```python
from build123d import *

# Parameters (mm, degrees)
ESQUISSE1_R        = 9.739786638
BOSS_EXTRU_1_DEPTH = 5.5
ESQUISSE2_R        = 9.739786638
ESQUISSE2_R_2      = 1.4
BOSS_EXTRU_2_DEPTH = 0.5
CHANFREIN1_SIZE    = 0.2
BOSS_EXTRU_3_START = -5.5
BOSS_EXTRU_3_DEPTH = 5.5
BOSS_EXTRU_4_START = 42
BOSS_EXTRU_4_DEPTH = 42
BOSS_EXTRU_5_DEPTH = 22
BOSS_EXTRU_6_DEPTH = 46.25
ESQUISSE7_W        = 6
ESQUISSE7_H        = 17.089185867
BOSS_EXTRU_7_DEPTH = 23


with BuildPart() as part:
    # Esquisse1 → Boss.-Extru.1 (new body)
    with BuildSketch(Plane.XY):
        with Locations((-10.25, -10)):
            Circle(ESQUISSE1_R)
        with BuildLine():
            Line((-5.751675839, -9.877200395), (-6.833750507, -9.782531128))
            Line((-6.833750507, -9.782531128), (-6.949445107, -9.126394451))
            Line((-6.949445107, -9.126394451), (-5.953521963, -8.661987862))
            ThreePointArc((-5.953521963, -8.661987862), (-6.006634107, -8.502052772), (-6.065697468, -8.344218516))
            Line((-6.065697468, -8.344218516), (-7.138261768, -8.631611254))
            Line((-7.138261768, -8.631611254), (-7.47139109, -8.054614344))
            Line((-7.47139109, -8.054614344), (-6.678798898, -7.262022153))
            ThreePointArc((-6.678798898, -7.262022153), (-6.782621037, -7.131675902), (-6.891198054, -7.005263035))
            Line((-6.891198054, -7.005263035), (-7.818046533, -7.654249327))
            Line((-7.818046533, -7.654249327), (-8.328430264, -7.225986526))
            Line((-8.328430264, -7.225986526), (-7.847635402, -6.194918616))
            ThreePointArc((-7.847635402, -6.194918616), (-7.988951343, -6.109285545), (-8.133315872, -6.028898352))
            Line((-8.133315872, -6.028898352), (-8.791112727, -6.968329619))
            Line((-8.791112727, -6.968329619), (-9.417191057, -6.740455742))
            Line((-9.417191057, -6.740455742), (-9.317216173, -5.597737589))
            ThreePointArc((-9.317216173, -5.597737589), (-9.478728542, -5.566588183), (-9.641271425, -5.541362369))
            Line((-9.641271425, -5.541362369), (-9.940094206, -6.656584169))
            Line((-9.940094206, -6.656584169), (-10.606352849, -6.656584169))
            Line((-10.606352849, -6.656584169), (-10.903477232, -5.547700874))
            ThreePointArc((-10.903477232, -5.547700874), (-11.065761738, -5.574558464), (-11.226956242, -5.607329229))
            Line((-11.226956242, -5.607329229), (-11.126406846, -6.756614081))
            Line((-11.126406846, -6.756614081), (-11.752485176, -6.984487958))
            Line((-11.752485176, -6.984487958), (-12.406540122, -6.050400691))
            ThreePointArc((-12.406540122, -6.050400691), (-12.550096477, -6.132241451), (-12.690551241, -6.219297732))
            Line((-12.690551241, -6.219297732), (-12.206963835, -7.256354271))
            Line((-12.206963835, -7.256354271), (-12.717347566, -7.684617071))
            Line((-12.717347566, -7.684617071), (-13.638885709, -7.039349117))
            ThreePointArc((-13.638885709, -7.039349117), (-13.74618945, -7.166864047), (-13.848697947, -7.298264801))
            Line((-13.848697947, -7.298264801), (-13.051434053, -8.095528695))
            Line((-13.051434053, -8.095528695), (-13.384563375, -8.672525605))
            Line((-13.384563375, -8.672525605), (-14.450903238, -8.3868007))
            ThreePointArc((-14.450903238, -8.3868007), (-14.508366703, -8.545244687), (-14.559856563, -8.705729393))
            Line((-14.559856563, -8.705729393), (-13.557961929, -9.172920534))
            Line((-13.557961929, -9.172920534), (-13.673656528, -9.829057211))
            Line((-13.673656528, -9.829057211), (-14.74934404, -9.923167674))
            ThreePointArc((-14.74934404, -9.923167674), (-14.749021481, -10.093838761), (-14.74222728, -10.264374865))
            Line((-14.74222728, -10.264374865), (-13.665452724, -10.358580432))
            Line((-13.665452724, -10.358580432), (-13.549758125, -11.014717109))
            Line((-13.549758125, -11.014717109), (-14.506309194, -11.460764198))
            ThreePointArc((-14.506309194, -11.460764198), (-14.447094307, -11.623083293), (-14.381691786, -11.78300953))
            Line((-14.381691786, -11.78300953), (-13.360941463, -11.509500306))
            Line((-13.360941463, -11.509500306), (-13.027812142, -12.086497216))
            Line((-13.027812142, -12.086497216), (-13.758807936, -12.817493011))
            ThreePointArc((-13.758807936, -12.817493011), (-13.646852578, -12.951506829), (-13.529782028, -13.081076086))
            Line((-13.529782028, -13.081076086), (-12.681156698, -12.486862233))
            Line((-12.681156698, -12.486862233), (-12.170772967, -12.915125033))
            Line((-12.170772967, -12.915125033), (-12.600738895, -13.837189942))
            ThreePointArc((-12.600738895, -13.837189942), (-12.448909121, -13.926168447), (-12.293716433, -14.009142444))
            Line((-12.293716433, -14.009142444), (-11.708090504, -13.172781941))
            Line((-11.708090504, -13.172781941), (-11.082012174, -13.400655818))
            Line((-11.082012174, -13.400655818), (-11.169878896, -14.404977051))
            ThreePointArc((-11.169878896, -14.404977051), (-10.996236031, -14.437694422), (-10.821442589, -14.463569577))
            Line((-10.821442589, -14.463569577), (-10.559109026, -13.48452739))
            Line((-10.559109026, -13.48452739), (-9.892850383, -13.48452739))
            Line((-9.892850383, -13.48452739), (-9.632173683, -14.457386077))
            ThreePointArc((-9.632173683, -14.457386077), (-9.45766281, -14.42969545), (-9.284373537, -14.395175256))
            Line((-9.284373537, -14.395175256), (-9.372796385, -13.384497479))
            Line((-9.372796385, -13.384497479), (-8.746718055, -13.156623602))
            Line((-8.746718055, -13.156623602), (-8.164782025, -13.987714383))
            ThreePointArc((-8.164782025, -13.987714383), (-8.010469052, -13.903139907), (-7.859580663, -13.812596936))
            Line((-7.859580663, -13.812596936), (-8.292239396, -12.884757289))
            Line((-8.292239396, -12.884757289), (-7.781855665, -12.456494489))
            Line((-7.781855665, -12.456494489), (-6.938532496, -13.046995729))
            ThreePointArc((-6.938532496, -13.046995729), (-6.822819391, -12.916236114), (-6.712266113, -12.78108593))
            Line((-6.712266113, -12.78108593), (-7.447769178, -12.045582865))
            Line((-7.447769178, -12.045582865), (-7.114639857, -11.468585954))
            Line((-7.114639857, -11.468585954), (-6.100183444, -11.740408731))
            ThreePointArc((-6.100183444, -11.740408731), (-6.036436962, -11.579837499), (-5.978900904, -11.416937723))
            Line((-5.978900904, -11.416937723), (-6.941241303, -10.968191026))
            Line((-6.941241303, -10.968191026), (-6.825546704, -10.312054348))
            Line((-6.825546704, -10.312054348), (-5.755303948, -10.21842024))
            ThreePointArc((-5.755303948, -10.21842024), (-5.750254354, -10.04784472), (-5.751675839, -9.877200395))
        make_face(mode=Mode.SUBTRACT)
    extrude(amount=BOSS_EXTRU_1_DEPTH)

    # Esquisse2 → Boss.-Extru.2 (add)
    with BuildSketch(Plane.XY.offset(5.5)):
        with Locations((-10.25, -10)):
            Circle(ESQUISSE2_R)
        with Locations((-10.249601616, -10.07055578)):
            Circle(ESQUISSE2_R_2, mode=Mode.SUBTRACT)
    extrude(amount=BOSS_EXTRU_2_DEPTH)

    # Chanfrein1
    chanfrein1_edges = [part.edges().sort_by_distance(p)[0] for p in [
        (-11.649601616, -10.07055578, 6),
    ]]
    chamfer(chanfrein1_edges, length=CHANFREIN1_SIZE)

    # Esquisse3 → Boss.-Extru.3 (add)
    with BuildSketch(Plane.XY.offset(6).offset(BOSS_EXTRU_3_START)):
        with BuildLine():
            Line((-10.25, -0.260213362), (39.75, -0.260213362))
            Line((39.75, -0.260213362), (39.75, -19.739786638))
            Line((39.75, -19.739786638), (-10.25, -19.739786638))
            ThreePointArc((-10.25, -19.739786638), (-19.989786638, -10), (-10.25, -0.260213362))
        make_face()
        with BuildLine():
            Line((33.837373972, -17.739786638), (-10.25, -17.739786638))
            ThreePointArc((-10.25, -17.739786638), (-17.989786638, -10), (-10.25, -2.260213362))
            Line((-10.25, -2.260213362), (33.837373972, -2.260213362))
            ThreePointArc((33.837373972, -2.260213362), (30.010213362, -10), (33.837373972, -17.739786638))
        make_face(mode=Mode.SUBTRACT)
    extrude(amount=BOSS_EXTRU_3_DEPTH)

    # Esquisse4 → Boss.-Extru.4 (add)
    with BuildSketch(Plane(origin=(0, 0, 0.5), x_dir=(-1, 0, 0), z_dir=(0, 0, -1)).offset(BOSS_EXTRU_4_START)):
        with BuildLine():
            Line((-39.75, -0.260213362), (-39.75, -19.739786638))
            ThreePointArc((-39.75, -19.739786638), (-30.010213362, -10), (-39.75, -0.260213362))
        make_face()
    extrude(amount=-BOSS_EXTRU_4_DEPTH)

    # Esquisse5 → Boss.-Extru.5 (add)
    with BuildSketch(Plane(origin=(39.75, 0, 0), x_dir=(0, 0, -1), z_dir=(1, 0, 0))):
        Polygon((34.25, -0.260213362), (34.25, -17.347570489), (39.5, -17.347570489), (41.5, -17.347570489), (41.5, -0.260213362), align=None)
    extrude(amount=BOSS_EXTRU_5_DEPTH)

    # Esquisse6 → Boss.-Extru.6 (add)
    with BuildSketch(Plane.XY.offset(-34.25)):
        Polygon((61.75, -0.260213362), (59.5, -0.260213362), (59.75, -17.347570489), (61.75, -17.347570489), align=None)
    extrude(amount=BOSS_EXTRU_6_DEPTH)

    # Esquisse7 → Boss.-Extru.7 (add)
    with BuildSketch(Plane(origin=(59.483460022, 0.870284673, 0), x_dir=(0, 0, 1), z_dir=(-0.9998929884849062, -0.014629134585590956, 0))):
        with Locations((9, -9.675211958)):
            Rectangle(ESQUISSE7_W, ESQUISSE7_H)
    extrude(amount=BOSS_EXTRU_7_DEPTH)


solid = part.part
```
Source: CAD feature listing. Evaluate the final solid. Frame: model axes, mm. A direction names the side the tool comes from. Coordinates: 2 decimals unless noted, no trailing zeros. Loops run counter-clockwise (first coordinate to the right, second up) from the corner with the lowest first, then second, coordinate; pieces in that order, holes last. Notation, with made-up numbers: (-15, -23) -> (-8, -23) arc R13 ccw to (-8, -6) -> close; hole circle Ø8 at (-0.75, -1.75). An arc over 180 degrees is marked (long way). One line per item, written item: value. Start each with the question number.
Q1. Section query B-B, the plane x = 5. Return the cut outline in (y, z), and give its area (3 significant figures).
Q2. Section query C-C, the plane z = -18. Return the cut outline in (x, y).
Q3. Section query D-D, the plane z = 4. Give the number of separate pieces and of enclosed holes in the cut face, and give its area (3 significant figures).
Q4. Set-up query: faces 4 (the face through (54, -17.348, -35)), 5 (the face through (-10, -14, 0)), 6 (the face through (15, -1, 0.5)). Return all of +Z, -Z, +X, -X, +Y, -Y with unobstructed straight access to the full face (end or side cutting, diameter ignored); none if empty.
Q5. Contact query for flat-ended pins moving along their axis: P1, Ø4.5, axis at x = -10.5, y = -9.5, coming from the -Z side; P2, Ø3, axis at x = 31, z = -19, coming from the +Y side; P3, Ø1, axis at x = 24.5, y = -1.5, coming from the -Z side; P4, Ø11, axis at x = 51.5, z = -15, coming from the -Y side. Output: stop coordinate, or through.
Q6. Section query A-A, the plane y = -3.25. Return the cut outline in (x, z), and give its area (3 significant figures).
Q7. Mould query, pull axis Z, two halves, no side actions, for faces 1 (the face through (50, -9, -34.25)), 2 (the face through (15, -19, 0.5)), 3 (the face through (15, -17.74, 3)). Classes: pulls with the +Z half, pulls with the -Z half, needs draft (parallel to the pull), parting line crosses it, or undercut.
Q8. Line query: line 1 along Y through (x, z) = (22.5, 5.5); line 2 along X through (y, z) = (-14.5, 4.5); line 3 along Z through (x, y) = (53.5, -4). Output: solid intervals per line, ascending.
Results:
1. outline: (-19.74, 0.5) -> (-17.74, 0.5) -> (-17.74, 6) -> (-19.74, 6) -> close; (-2.26, 0.5) -> (-0.26, 0.5) -> (-0.26, 6) -> (-2.26, 6) -> close
1. area: 22.0 mm^2
2. outline: (39.75, -19.74) -> (39.75, -0.26) arc R9.74 ccw to start; (59.5, -0.26) -> (59.75, -17.35) -> (61.75, -17.35) -> (61.75, -0.26) -> close
3. separate pieces: 2
3. enclosed holes: 2
3. area: 606 mm^2
4. face 4: -Z, +X, -Y
4. face 5: -Z, -X, +Y, -Y
4. face 6: -Z, +Y
5. P1: z = 5.5
5. P2: y = -3.5
5. P3: z = 0.5
5. P4: through
6. outline: (-17.27, 0) -> (-3.23, 0) -> (-3.23, 6) -> (-17.27, 6) -> close; (32.73, -41.5) -> (61.75, -41.5) -> (61.75, 12) -> (36.54, 12) -> (36.54, 6) -> (32.73, 6) -> close; hole (39.75, -34.25) -> (59.54, -34.25) -> (59.54, 6) -> (39.75, 6) -> close
6. area: 817 mm^2
7. face 1: undercut
7. face 2: pulls with the -Z half
7. face 3: needs draft
8. line 1: -19.74 to -17.74, -2.26 to -0.26
8. line 2: -18.89 to -1.61, 31.11 to 39.75, 59.71 to 61.75
8. line 3: -41.5 to -34.25, 6 to 12
